Part model, mm, in its own coordinate system. Face numbers are marked on the shaded views. A direction names the side the tool comes from. Round coordinates to 2 decimals unless told otherwise and drop trailing zeros. Order: outer loops, then holes, each group sorted by start corner. A loop starts at its lowest first (then second) coordinate and runs counter-clockwise, first axis right, second up. Notation, with made-up numbers: M 29,3.5 L 60,3.5 A21 cw 60,17.5 Z; hole C -20.5,56 d4. An arc over 180 degrees is marked long. Write each question's results on one line, items separated by ' | '. Start each with the question number.
1. Drop flat-ended pins along their axis: pin 1 Ø0.6 at (x, z) = (6.5, 75.5) entering from +Y; pin 2 Ø2.5 at (x, z) = (-4, 78.5) entering from +Y; pin 3 Ø2.5 at (x, y) = (10.5, 8) entering from +Z. Give the stop position or say it passes through.
2. Band-saw the part on B-B, the plane x = 29. List the corners of the cut face in (y, z), then the cut area to 3 significant figures.
3. Probe L1, parallel to X at y = 8, z = 75.65; L2, parallel to Z at x = -7.5, y = 1; L3, parallel to Z at x = -29.5, y = 6.25. List the from-to ranges inside material, lowest first. Write a range as [from, to].
4. Band-saw the part on A-A, the plane z = 75.25. List the corners of the cut face in (x, y), then the cut area to 3 significant figures.
5. Which spindle directions (+Z, -Z, +X, -X, +Y, -Y) get a long thin tool onto all of the face, cutting with end or side? Do the marked faces 1, 2 and 3. Say none if no direction does.
```python
from build123d import *

# Parameters (mm, degrees)
F0_R     = 1.25
F1_DEPTH = 3
F2_W     = 72
F2_H     = 2
F3_DEPTH = 4
F5_DEPTH = 3


with BuildPart() as f1:
    # F0 (on Front) → F1 (new body)
    with BuildSketch(Plane.XZ):
        with BuildLine():
            Line((33.312092313, 76.6384017421), (-25.687907687, 76.6384017421))
            Line((-25.687907687, 76.6384017421), (-31.1261699955, 76.6384017421))
            ThreePointArc((-31.1261699955, 76.6384017421), (-30.6147865133, 75.6959584788), (-30.437907687, 74.6384017421))
            Line((-30.437907687, 74.6384017421), (33.312092313, 74.6384017421))
            Line((33.312092313, 74.6384017421), (33.312092313, 76.6384017421))
        make_face()
        with BuildLine():
            ThreePointArc((-30.437907687, 74.6384017421), (-30.6147865133, 75.6959584788), (-31.1261699955, 76.6384017421))
            Line((-31.1261699955, 76.6384017421), (-36.2496453785, 76.6384017421))
            ThreePointArc((-36.2496453785, 76.6384017421), (-36.6087380484, 73.2131824607), (-33.687907687, 71.3884017421))
            ThreePointArc((-33.687907687, 71.3884017421), (-32.2626884057, 71.7175713807), (-31.1261699955, 72.6384017421))
            ThreePointArc((-31.1261699955, 72.6384017421), (-30.6147865133, 73.5808450054), (-30.437907687, 74.6384017421))
        make_face()
        with Locations((-33.687907687, 74.6384017421)):
            Circle(F0_R, mode=Mode.SUBTRACT)
        with BuildLine():
            ThreePointArc((-33.687907687, 71.3884017421), (-36.6087380484, 73.2131824607), (-36.2496453785, 76.6384017421))
            Line((-36.2496453785, 76.6384017421), (-38.687907687, 76.6384017421))
            Line((-38.687907687, 76.6384017421), (-38.687907687, 71.3884017421))
            Line((-38.687907687, 71.3884017421), (-33.687907687, 71.3884017421))
        make_face()
        with BuildLine():
            Line((-31.1261699955, 76.6384017421), (-25.687907687, 76.6384017421))
            Line((-25.687907687, 76.6384017421), (33.312092313, 76.6384017421))
            Line((33.312092313, 76.6384017421), (33.312092313, 79.6384017421))
            Line((33.312092313, 79.6384017421), (-38.687907687, 79.6384017421))
            Line((-38.687907687, 79.6384017421), (-38.687907687, 76.6384017421))
            Line((-38.687907687, 76.6384017421), (-36.2496453785, 76.6384017421))
            ThreePointArc((-36.2496453785, 76.6384017421), (-33.687907687, 77.8884017421), (-31.1261699955, 76.6384017421))
        make_face()
        with BuildLine():
            Line((-36.2496453785, 76.6384017421), (-31.1261699955, 76.6384017421))
            ThreePointArc((-31.1261699955, 76.6384017421), (-33.687907687, 77.8884017421), (-36.2496453785, 76.6384017421))
        make_face()
    extrude(amount=-F1_DEPTH)

    # F2 (on face) → F3 (join)
    with BuildSketch(Plane(origin=(0, 3, 0), x_dir=(-1, 0, 0), z_dir=(0, 1, 0))):
        with Locations((2.687907687, 75.6384017421)):
            Rectangle(F2_W, F2_H)
    extrude(amount=F3_DEPTH)

    # F4 (on face) → F5 (join)
    with BuildSketch(Plane.XY.offset(76.6384017421)):
        with BuildLine():
            Line((-38.687907687, 7), (-34.7851954552, 7))
            ThreePointArc((-34.7851954552, 7), (-34.3208407412, 9.9121323176), (-31.692866236, 11.25))
            Line((-31.692866236, 11.25), (-38.687907687, 11.25))
            Line((-38.687907687, 11.25), (-38.687907687, 7))
        make_face()
        with BuildLine():
            ThreePointArc((-32.442866236, 7), (-32.2518832303, 9.1180339887), (-30.442866236, 8))
            ThreePointArc((-30.442866236, 8), (-30.5748322472, 7.4409830056), (-30.942866236, 7))
            Line((-30.942866236, 7), (-28.6005370168, 7))
            ThreePointArc((-28.6005370168, 7), (-28.4825259143, 7.4938231349), (-28.442866236, 8))
            ThreePointArc((-28.442866236, 8), (-29.3947691971, 10.2980970389), (-31.692866236, 11.25))
            ThreePointArc((-31.692866236, 11.25), (-34.3208407412, 9.9121323176), (-34.7851954552, 7))
            Line((-34.7851954552, 7), (-32.442866236, 7))
        make_face()
        with BuildLine():
            ThreePointArc((-30.942866236, 7), (-31.692866236, 6.75), (-32.442866236, 7))
            Line((-32.442866236, 7), (-34.7851954552, 7))
            ThreePointArc((-34.7851954552, 7), (-31.692866236, 4.75), (-28.6005370168, 7))
            Line((-28.6005370168, 7), (-30.942866236, 7))
        make_face()
    extrude(amount=-F5_DEPTH)


solid = f1.part
```
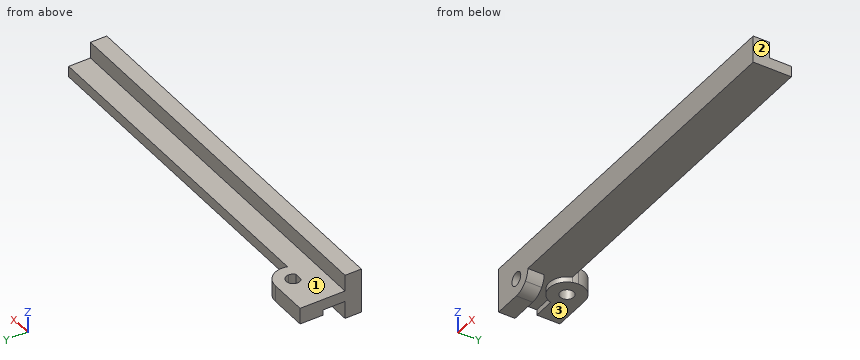
Solution:
1) pin 1: y = 7 | pin 2: y = 3 | pin 3: z = 76.64
2) outline: M 0,74.64 L 7,74.64 L 7,76.64 L 3,76.64 L 3,79.64 L 0,79.64 Z | area: 23.0 mm^2
3) L1: [-38.69, -32.94], [-30.44, -28.44] | L2: [74.64, 79.64] | L3: [73.64, 76.64]
4) outline: M -38.69,0 L -34.78,0 L -34.78,3 L -32.6,3 L -32.6,0 L 33.31,0 L 33.31,7 L -28.6,7 A3.25 ccw -31.69,11.25 L -38.69,11.25 Z; hole M -32.44,7 L -30.94,7 A1.25 ccw long Z | area: 534 mm^2
5) face 1: +Z, +X, -X, +Y | face 2: +Z, -Z, +X, +Y, -Y | face 3: -Z, +X, -X, +Y
